```python
from build123d import *

# Parameters (mm, degrees)
F0_R      = 8.9296875
F0_R_2    = 3.96875
F0_R_3    = 3.175
F0_R_4    = 1.68671875
F1_DEPTH  = 3.175
F2_DEPTH  = 1.3208
F3_DEPTH  = 6.0833
F1_FACE_R = 8.9296875


# Not quite as in the source:
# - a length typed as a fraction of an inch, garbled in the dataset ("3 / 203.2 mm" for 3/8 in), is restored


with BuildPart() as f1:
    # F0 (on Top) → F1 (new body)
    with BuildSketch(Plane.XY):
        Circle(F0_R)
        Circle(F0_R_2, mode=Mode.SUBTRACT)
        Circle(F0_R_2)
        Circle(F0_R_3, mode=Mode.SUBTRACT)
        Circle(F0_R_3)
        Circle(F0_R_4, mode=Mode.SUBTRACT)
        Circle(F0_R_4)
    extrude(amount=-F1_DEPTH)

    # F0 (on Top) → F2 (join)
    with BuildSketch(Plane.XY):
        Circle(F0_R_2)
        Circle(F0_R_3, mode=Mode.SUBTRACT)
        Circle(F0_R_3)
        Circle(F0_R_4, mode=Mode.SUBTRACT)
        Circle(F0_R_4)
    extrude(amount=F2_DEPTH)

    # F0 (on Top) → F3 (join)
    with BuildSketch(Plane.XY):
        Circle(F0_R_3)
        Circle(F0_R_4, mode=Mode.SUBTRACT)
    extrude(amount=F3_DEPTH)

    # F1_face (on face) → F4 section 0
    with BuildSketch(Plane(origin=(0, 0, -3.175), x_dir=(1, 0, 0), z_dir=(0, 0, -1)), mode=Mode.PRIVATE) as f4_s0:
        Circle(F1_FACE_R)
    loft([f4_s0.sketch, Vertex(0, 0, 0)], mode=Mode.SUBTRACT)


solid = f1.part
```
Work out the finished part from the listing and answer in its coordinate system (mm). A direction names the side the tool comes from. Coordinates: 2 decimals unless noted, no trailing zeros. Loops run counter-clockwise (first coordinate to the right, second up) from the corner with the lowest first, then second, coordinate; pieces in that order, holes last.
1) For faces 1 (the cylindrical face through (-1.243, 1.14, 3.669)), 2 (the conical face through (0, 0, 0)), determine the directions among +Z, -Z, +X, -X, +Y, -Y from which every point of the face is accessible in a straight line to the end or side of a thin tool.
Results:
face 1: +Z
face 2: -Z
2) Section B-B (z = 1) is taken. Give the vertices of the cut face in (x, y).
Results:
outline: circle Ø7.94 at (0, 0)
3) For a pull along X with two mould halves and no side action, classify faces 3 (the flat face through (0, 0, 1.321)), 4 (the cylindrical face through (-0.69, -3.1, 3.67)), 5 (the flat face through (2, -4, 0)) as +X half, -X half, draft (parallel to the pull), parting line (faces both ways), or undercut.
Results:
face 3: undercut
face 4: parting line
face 5: draft
4) Flat-ended cylindrical pins translate along their axes: pin 1 (10 mm diameter, centred on x = -2.5, y = -1, fed in from -Z); pin 2 (4 mm diameter, centred on x = -5.5, z = 0, fed in from +Y); pin 3 (10 mm diameter, centred on x = -1.5, y = -1.5, fed in from -Z); pin 4 (3.5 mm diameter, centred on x = 0.5, y = -0.5, fed in from +Z). Find the tip coordinate at first contact, or state that the pin passes through.
Results:
pin 1: stops at z = -2.74
pin 2: stops at y = 8.22
pin 3: stops at z = -2.53
pin 4: stops at z = 6.08
5) Section A-A (z = 4) is taken. Give the vertices of the cut face in (x, y) (3 decimals), plus the area to 3 significant figures.
Results:
outline: circle Ø6.35 at (0, 0); hole circle Ø3.373 at (0, 0)
area: 22.7 mm2
6) Consider probe 1 along Y at (x, z) = (0, 3.8) (3 decimals); probe 2 along Z at (x, y) = (8, -3.25). Determine where each line is inside the solid, lowest interval first.
Results:
probe 1: y = -3.175 to -1.687, 1.687 to 3.175
probe 2: z = -3.07 to 0
7) Section C-C (z = -1.25) is taken. Give the vertices of the cut face in (x, y), plus the area to 3 significant figures.
Results:
outline: circle Ø17.86 at (0, 0); hole circle Ø7.03 at (0, 0)
area: 212 mm2
